Here's how the part is built. I have some questions about the finished solid (model axes, mm). Coordinates: 2 decimals unless noted, no trailing zeros. Order: outer loops, then holes, each group sorted by start corner. A loop starts at its lowest first (then second) coordinate and runs counter-clockwise, first axis right, second up. Notation, with made-up numbers: (59, -2.75) - (106, -2.75) arc R28 ccw to (106, 17.25) - close; hole circle Ø8 at (4, 64). An arc over 180 degrees is marked (long way). Answer as CSV lines item,"result". Start each with the question number.
Item 1: Imagine slicing it at B-B on x = -71. List the corners of the cut face in (y, z) for me, and give its area (3 significant figures).
Item 2: I'm going to push flat-ended pins straight in: pin 1 (2.5 mm diameter, centred on x = -80, y = 36, fed in from +Z); pin 2 (4 mm diameter, centred on x = -75, y = -52.5, fed in from -Z). Where does each tip first touch, or does it pass through?
Item 3: I need wall thicknesses on line 1 (Y direction, x = -52.5, z = 0.75); line 2 (Y direction, x = -87.5, z = 1); line 3 (Y direction, x = -56, z = 1.15). Which ranges of each line are inside material? Lowest first, please.
Item 4: Imagine slicing it at C-C on z = 0.75. Count the separate pieces of the cut face and the enclosed holes in it, and give its area (3 significant figures).
Item 5: Imagine slicing it at D-D on y = 30. List the corners of the cut face in (x, z) for me, and give its area (3 significant figures).
Item 6: Imagine slicing it at A-A on y = -36. List the corners of the cut face in (x, z) for me.
from build123d import *

# Parameters (mm, degrees)
SKETCH1_R          = 1.6
EXTRUDE1_DEPTH     = 3
SKETCH2_R          = 1.6
CUT_EXTRUDE1_DEPTH = 26
SKETCH3_R          = 2.75
CUT_EXTRUDE2_DEPTH = 10


with BuildPart() as part:
    # Sketch1 → Extrude1 (new body)
    with BuildSketch(Plane.XY):
        Polygon((-95, 62.5), (-95, -62.5), (-55, -62.5), (-45, -62.5), (-45, -42.5), (-55, -42.5), (-75, -22.5), (-75, 22.5), (-55, 42.5), (-45, 42.5), (-45, 62.5), (-55, 62.5), align=None)
        with Locations((-55, -52.5)):
            Circle(SKETCH1_R, mode=Mode.SUBTRACT)
        with Locations((-75, -52.5)):
            Circle(SKETCH1_R, mode=Mode.SUBTRACT)
        with Locations((-55, 52.5)):
            Circle(SKETCH1_R, mode=Mode.SUBTRACT)
        with Locations((-75, 52.5)):
            Circle(SKETCH1_R, mode=Mode.SUBTRACT)
    extrude(amount=EXTRUDE1_DEPTH)

    # Sketch2 → Cut-Extrude1 (cut)
    with BuildSketch(Plane.XY.offset(3)):
        with Locations((-80, 36)):
            Circle(SKETCH2_R)
        with Locations((-90, 36)):
            Circle(SKETCH2_R)
        with Locations((-80, -36)):
            Circle(SKETCH2_R)
        with Locations((-90, -36)):
            Circle(SKETCH2_R)
    extrude(amount=-CUT_EXTRUDE1_DEPTH, mode=Mode.SUBTRACT)

    # Sketch3 → Cut-Extrude2 (cut)
    with BuildSketch(Plane(origin=(0, 0, 0), x_dir=(-1, 0, 0), z_dir=(0, 0, -1))):
        with Locations((87.5, 55)):
            Circle(SKETCH3_R)
        with Locations((87.5, 30)):
            Circle(SKETCH3_R)
        with Locations((87.5, -30)):
            Circle(SKETCH3_R)
        with Locations((87.5, -55)):
            Circle(SKETCH3_R)
    extrude(amount=-CUT_EXTRUDE2_DEPTH, mode=Mode.SUBTRACT)


solid = part.part
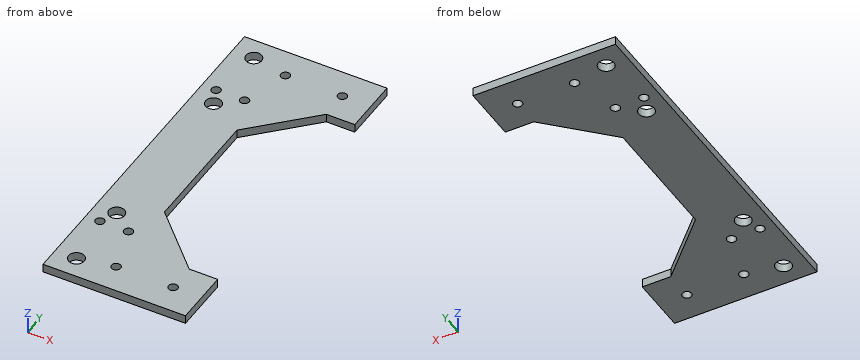
Responses:
1,outline,"(-62.5, 0) - (-26.5, 0) - (-26.5, 3) - (-62.5, 3) - close; (26.5, 0) - (62.5, 0) - (62.5, 3) - (26.5, 3) - close"
1,area,"216 mm^2"
2,pin 1,"passes through"
2,pin 2,"stops at z = 0"
3,line 1,"y = -62.5 to -42.5, 42.5 to 62.5"
3,line 2,"y = -62.5 to -57.75, -52.25 to -32.75, -27.25 to 27.25, 32.75 to 52.25, 57.75 to 62.5"
3,line 3,"y = -62.5 to -53.75, -51.25 to -41.5, 41.5 to 51.25, 53.75 to 62.5"
4,separate pieces,"1"
4,enclosed holes,"12"
4,area,"3,940 mm^2"
5,outline,"(-95, 0) - (-90.25, 0) - (-90.25, 3) - (-95, 3) - close; (-84.75, 0) - (-67.5, 0) - (-67.5, 3) - (-84.75, 3) - close"
5,area,"66.0 mm^2"
6,outline,"(-95, 0) - (-91.6, 0) - (-91.6, 3) - (-95, 3) - close; (-88.4, 0) - (-81.6, 0) - (-81.6, 3) - (-88.4, 3) - close; (-78.4, 0) - (-61.5, 0) - (-61.5, 3) - (-78.4, 3) - close"
